The listing builds one solid part. Answer for the finished solid, in the listing's coordinates (mm). Face numbers are marked on the shaded views. A direction names the side the tool comes from. Round coordinates to 2 decimals unless told otherwise and drop trailing zeros. Order: outer loops, then holes, each group sorted by start corner. A loop starts at its lowest first (then second) coordinate and runs counter-clockwise, first axis right, second up. Notation, with made-up numbers: (7, -31) -> (14, -31) arc R13 ccw to (14, -12) -> close; hole circle Ø7 at (0.25, -38). An arc over 180 degrees is marked (long way). Answer in a Markdown table with one row per item. Add a question column.
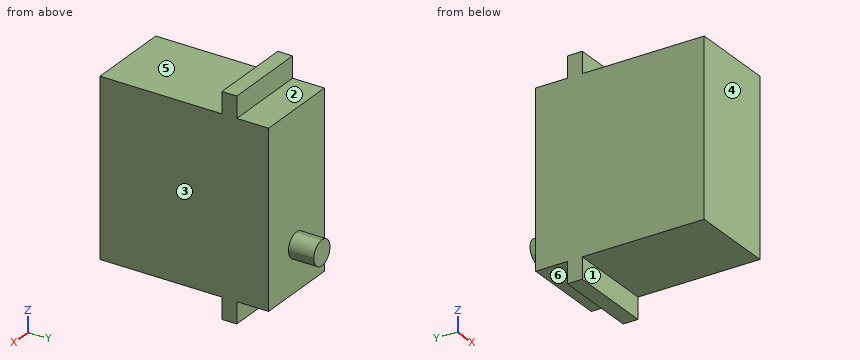
```python
from build123d import *

# Parameters (mm, degrees)
SKETCH2_W           = 41
SKETCH2_H           = 39.75
SKETCH2_W_2         = 5
SKETCH2_H_2         = 3.5
SKETCH2_W_3         = 5.8
SKETCH2_H_3         = 6
BOSS_EXTRUDE1_DEPTH = 20.1
CUT_EXTRUDE1_DEPTH  = 6


with BuildPart() as part:
    # Sketch2 → Boss-Extrude1 (new body)
    with BuildSketch(Plane(origin=(0, 0, 0), x_dir=(0, 0, -1), z_dir=(1, 0, 0))):
        Rectangle(SKETCH2_W, SKETCH2_H)
        with Locations((-23, 10.625)):
            Rectangle(SKETCH2_W_2, SKETCH2_H_2)
        with Locations((10.1, 22.875)):
            Rectangle(SKETCH2_W_3, SKETCH2_H_3)
        with Locations((23, 10.625)):
            Rectangle(SKETCH2_W_2, SKETCH2_H_2)
    extrude(amount=BOSS_EXTRUDE1_DEPTH)

    # Sketch3 → Cut-Extrude1 (cut)
    with BuildSketch(Plane(origin=(0, 19.875, 0), x_dir=(1, 0, 0), z_dir=(0, 1, 0))):
        with BuildLine():
            Line((10.05, 7.2), (12.95, 7.2))
            Line((12.95, 7.2), (12.95, 10.1))
            ThreePointArc((12.95, 10.1), (12.100609665, 8.049390335), (10.05, 7.2))
        make_face()
        with BuildLine():
            ThreePointArc((10.05, 13), (12.100609665, 12.150609665), (12.95, 10.1))
            Line((12.95, 10.1), (12.95, 13))
            Line((12.95, 13), (10.05, 13))
        make_face()
        with BuildLine():
            ThreePointArc((7.15, 10.1), (7.999390335, 12.150609665), (10.05, 13))
            Line((10.05, 13), (7.15, 13))
            Line((7.15, 13), (7.15, 10.1))
        make_face()
        with BuildLine():
            Line((7.15, 7.2), (10.05, 7.2))
            ThreePointArc((10.05, 7.2), (7.999390335, 8.049390335), (7.15, 10.1))
            Line((7.15, 10.1), (7.15, 7.2))
        make_face()
        Polygon((0, 7.2), (7.15, 7.2), (7.15, 10.1), (7.15, 13), (0, 13), align=None)
        Polygon((12.95, 7.2), (20.1, 7.2), (20.1, 13), (12.95, 13), (12.95, 10.1), align=None)
    extrude(amount=CUT_EXTRUDE1_DEPTH, mode=Mode.SUBTRACT)


solid = part.part
```
Item 1: The part is cut by section C-C, the plane y = 17.5. Give the vertices of the cut face in (x, z).
Item 2: Flat-ended cylindrical pins translate along their axes: P1, Ø1.5, axis at x = 10.5, z = 22.5, coming from the +Y side (3 decimals); P2, Ø3, axis at x = 14.5, z = 17, coming from the +Y side (3 decimals); P3, Ø8, axis at x = 5.5, y = 20.5, coming from the +Z side. Find the tip coordinate at first contact, or state that the pin passes through.
Item 3: For a pull along Z with two mould halves and no side action, classify the marked faces 4, 5 and 6 as released by +Z, released by -Z, zero draft, split by the parting line, or undercut.
Item 4: The part is cut by section A-A, the plane x = 15. Give the vertices of the cut face in (y, z) (3 decimals).
Item 5: The part is cut by section D-D, the plane x = 8. Give the vertices of the cut face in (y, z) (3 decimals).
Item 6: The part is cut by section B-B, the plane z = 7.5. Give the vertices of the cut face in (x, y) (3 decimals), and give its area (3 significant figures).
Item 7: A tool of negligible diameter and unlimited length cuts with its end or side. For the marked faces 1, 2 and 3, from which of +Z, -Z, +X, -X, +Y, -Y can it reach the whole face along a straight path? Write none if from no direction.
Item 8: Find the intervals of material crossed by probe 1 along Y at (x, z) = (4, -11.5) (3 decimals); probe 2 along Z at (x, y) = (15.5, -15.5); probe 3 along Y at (x, z) = (14.25, 23) (3 decimals), in increasing order. Write a range as [from, to].
Resolved:
| question | item | result |
|---|---|---|
| 1 | outline | (0, -20.5) -> (20.1, -20.5) -> (20.1, 20.5) -> (0, 20.5) -> close |
| 2 | P1 | y = 12.375 |
| 2 | P2 | y = 19.875 |
| 2 | P3 | z = 20.5 |
| 3 | face 4 | zero draft |
| 3 | face 5 | released by +Z |
| 3 | face 6 | released by -Z |
| 4 | outline | (-19.875, -20.5) -> (8.875, -20.5) -> (8.875, -25.5) -> (12.375, -25.5) -> (12.375, -20.5) -> (19.875, -20.5) -> (19.875, 20.5) -> (12.375, 20.5) -> (12.375, 25.5) -> (8.875, 25.5) -> (8.875, 20.5) -> (-19.875, 20.5) -> close |
| 5 | outline | (-19.875, -20.5) -> (8.875, -20.5) -> (8.875, -25.5) -> (12.375, -25.5) -> (12.375, -20.5) -> (19.875, -20.5) -> (19.875, -12.151) -> (25.875, -12.151) -> (25.875, -8.049) -> (19.875, -8.049) -> (19.875, 20.5) -> (12.375, 20.5) -> (12.375, 25.5) -> (8.875, 25.5) -> (8.875, 20.5) -> (-19.875, 20.5) -> close |
| 6 | outline | (0, -19.875) -> (20.1, -19.875) -> (20.1, 19.875) -> (0, 19.875) -> close |
| 6 | area | 799 mm2 |
| 7 | face 1 | -Z, +X, -X, -Y |
| 7 | face 2 | +Z, +X, -X, +Y |
| 7 | face 3 | +Z, -Z, +X, +Y, -Y |
| 8 | probe 1 | [-19.875, 19.875] |
| 8 | probe 2 | [-20.5, 20.5] |
| 8 | probe 3 | [8.875, 12.375] |
